Can you work these out from the model? Positions are in its coordinate system, mm. A direction names the side the tool comes from. Round coordinates to 2 decimals unless told otherwise and drop trailing zeros. Order: outer loops, then holes, each group sorted by start corner. A loop starts at its lowest first (then second) coordinate and runs counter-clockwise, first axis right, second up.
from build123d import *

# Parameters (mm, degrees)
SKETCH1_W           = 3
SKETCH1_H           = 10
SKETCH1_R           = 1.5
BOSS_EXTRUDE1_DEPTH = 3


with BuildPart() as part:
    # Sketch1 → Boss-Extrude1 (new body)
    # profile 1 of 2: a face of its own
    with BuildSketch(Plane(origin=(0, 0, 0), x_dir=(1, 0, 0), z_dir=(0, 1, 0))):
        Polygon((-90, 0), (-72.5, 0), (-72.5, -3), (-62.5, -3), (-62.5, 0), (-46.5, 0), (-46.5, 3.1), (-47.8, 3.1), (-47.8, 5.6), (-46.5, 5.6), (-46.5, 9.4), (-45, 9.4), (-45, 73), (-90, 73), align=None)
        with Locations((-84.5, 20)):
            Rectangle(SKETCH1_W, SKETCH1_H, mode=Mode.SUBTRACT)
        with Locations(Location((-84.5, 36.5, 0), (0, 0, 270))):
            Circle(SKETCH1_R, mode=Mode.SUBTRACT)
        with Locations((-84.5, 53)):
            Rectangle(SKETCH1_W, SKETCH1_H, mode=Mode.SUBTRACT)
    # profile 2 of 2: a face of its own
    with BuildSketch(Plane(origin=(0, 0, 0), x_dir=(1, 0, 0), z_dir=(0, 1, 0))):
        Polygon((0, 73), (-45, 73), (-45, 9.4), (-43.5, 9.4), (-43.5, 5.6), (-42.2, 5.6), (-42.2, 3.1), (-43.5, 3.1), (-43.5, 0), (-27.5, 0), (-27.5, -3), (-17.5, -3), (-17.5, 0), (0, 0), align=None)
        with Locations((-5.5, 20)):
            Rectangle(SKETCH1_W, SKETCH1_H, mode=Mode.SUBTRACT)
        with Locations(Location((-5.5, 36.5, 0), (0, 0, 270))):
            Circle(SKETCH1_R, mode=Mode.SUBTRACT)
        with Locations((-5.5, 53)):
            Rectangle(SKETCH1_W, SKETCH1_H, mode=Mode.SUBTRACT)
    extrude(amount=BOSS_EXTRUDE1_DEPTH)


solid = part.part
(1) I want a section at B-B, the plane x = -84.5. List the corners of the cut face in (y, z) for me, plus the area to 3 significant figures.
(2) Please list where these lines run through material, in increasing order: probe 1 along Z at (x, y) = (-84.5, 1.05); probe 2 along X at (y, z) = (0.65, -52); probe 3 along X at (y, z) = (1, -4).
(3) I want a section at D-D, the plane y = 0.9. Give the number of separate pieces and of enclosed holes in the cut face, plus the area to 3 significant figures.
(4) On a 3-axis mill with a long thin cutter (end or side, diameter ignored), from which of +Z, -Z, +X, -X, +Y, -Y can I reach the whole of each face in a straight line? I mean faces 1 (the face through (-6, 1, -25)), 2 (the face through (-23, 1, 3)), 3 (the face through (-36, 1, 0)). Say none if no direction works.
(5) I want a section at C-C, the plane z = -36.5. List the corners of the cut face in (x, y) for me.
(6) I want a section at A-A, the plane z = -7.5. List the corners of the cut face in (x, y) for me, plus the area to 3 significant figures.
(7) If we mould it in two halves opening along X, with no side actions, what happens to faces 4 (the face through (-46, 0, -36)), 5 (the face through (-17.5, 1, 2)), 6 (the face through (-72.5, 1, 1)), 7 (the face through (-43.5, 1, -8))? For each: pulls with the +X half, pulls with the -X half, needs draft (parallel to the pull), parting line crosses it, or undercut.
Ans:
1. outline: (0, -73) - (3, -73) - (3, -58) - (0, -58) - close; (0, -48) - (3, -48) - (3, -38) - (0, -38) - close; (0, -35) - (3, -35) - (3, -25) - (0, -25) - close; (0, -15) - (3, -15) - (3, 0) - (0, 0) - close
1. area: 150 mm2
2. probe 1: z = -73 to -58, -48 to -38, -35 to -25, -15 to 0
2. probe 2: x = -90 to -86, -83 to -7, -4 to 0
2. probe 3: x = -90 to -47.8, -42.2 to 0
3. separate pieces: 1
3. enclosed holes: 6
3. area: 6,460 mm2
4. face 1: +Y, -Y
4. face 2: +Z, +X, -X, +Y, -Y
4. face 3: +Z, +Y, -Y
5. outline: (-90, 0) - (-86, 0) - (-86, 3) - (-90, 3) - close; (-83, 0) - (-7, 0) - (-7, 3) - (-83, 3) - close; (-4, 0) - (0, 0) - (0, 3) - (-4, 3) - close
6. outline: (-90, 0) - (-46.5, 0) - (-46.5, 3) - (-90, 3) - close; (-43.5, 0) - (0, 0) - (0, 3) - (-43.5, 3) - close
6. area: 261 mm2
7. face 4: needs draft
7. face 5: pulls with the +X half
7. face 6: pulls with the -X half
7. face 7: undercut
